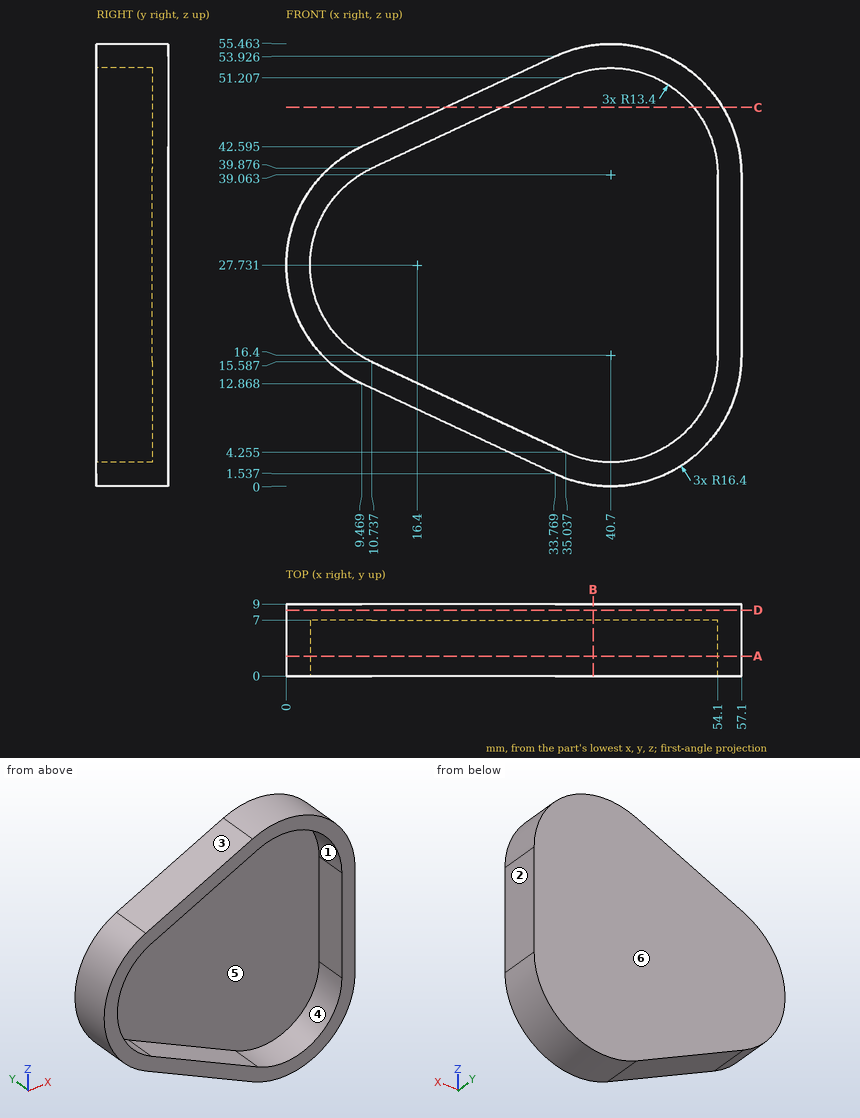
Answer from the drawing. Dimensions are ordinates in mm from the lowest x, y and z of the part. A direction names the side the tool comes from. Give positions to 0.01 mm unless a question says otherwise; leave off trailing zeros. Order: outer loops, then holes, each group sorted by start corner. A loop starts at its lowest first (then second) coordinate and runs counter-clockwise, first axis right, second up.
Item 1: For a pull along Z with two mould halves and no side action, classify the marked faces 3, 4, 5 and 6 as pulls with the +Z half, pulls with the -Z half, needs draft (parallel to the pull), parting line crosses it, or undercut.
From the geometry:
face 3: pulls with the +Z half
face 4: undercut
face 5: undercut
face 6: needs draft
Item 2: The part is cut by section B-B, the plane x = 38.5. Give the vertices of the cut face in (y, z) (1 decimal).
From the geometry:
outline: (0, 0.1) - (9, 0.1) - (9, 55.3) - (0, 55.3) - (0, 52.3) - (7, 52.3) - (7, 3.2) - (0, 3.2) - close
Item 3: The part is cut by section C-C, the plane z = 47.5. Give the vertices of the cut face in (x, y), and give its area (3 significant figures).
From the geometry:
outline: (19.99, 0) - (27.09, 0) - (27.09, 7) - (51.11, 7) - (51.11, 0) - (54.76, 0) - (54.76, 9) - (19.99, 9) - close
area: 145 mm2
Item 4: The part is cut by section D-D, the plane y = 8.25. Give the vertices of the cut face in (x, z) (1 decimal), and give its area (3 significant figures).
From the geometry:
outline: (9.5, 12.9) - (33.8, 1.5) arc R16.4 ccw to (57.1, 16.4) - (57.1, 39.1) arc R16.4 ccw to (33.8, 53.9) - (9.5, 42.6) arc R16.4 ccw to start
area: 2,370 mm2
Item 5: The part is cut by section A-A, the plane y = 2.5. Give the vertices of the cut face in (x, z) (1 decimal).
From the geometry:
outline: (9.5, 12.9) - (33.8, 1.5) arc R16.4 ccw to (57.1, 16.4) - (57.1, 39.1) arc R16.4 ccw to (33.8, 53.9) - (9.5, 42.6) arc R16.4 ccw to start; hole (10.7, 15.6) - (35, 4.3) arc R13.4 ccw to (54.1, 16.4) - (54.1, 39.1) arc R13.4 ccw to (35, 51.2) - (10.7, 39.9) arc R13.4 ccw to start
Item 6: Given pin 1 Ø4 at (x, y) = (44, 3) entering from -Z; pin 2 Ø1.5 at (x, y) = (37.5, 4) entering from -Z, each flat-ended and moving along its own axis, determine where each tip first touches the part or whether it passes through.
From the geometry:
pin 1: stops at z = 0.05
pin 2: stops at z = 0.18
Item 7: Which of the six approach directions +Z, -Z, +X, -X, +Y, -Y give full straight-line access (tool end or side, diameter ignored) to the marked faces 1 and 2?
From the geometry:
face 1: -Y
face 2: +Z, -Z, +X, +Y, -Y
Item 8: Find the intervals of material crossed by probe 1 along Y at (x, z) = (49, 21.5); probe 2 along Z at (x, y) = (8, 1) (1 decimal); probe 3 along Z at (x, y) = (18, 5), in increasing order.
From the geometry:
probe 1: y = 7 to 9
probe 2: z = 13.6 to 17.3, 38.2 to 41.8
probe 3: z = 8.89 to 12.2, 43.26 to 46.57
